Model file for the job. Use its own axes, mm. Give positions to 0.01 mm unless a question says otherwise; leave off trailing zeros. Write each loop counter-clockwise with the first axis right and the second up, starting at its lowest first coordinate (ties: lowest second). Pieces come first, ordered by that corner, then holes. Notation, with made-up numbers: (-2, -15) - (25, -15) arc R27 cw to (25, 16) - close; hole circle Ø2 at (65.25, 16). An arc over 180 degrees is marked (long way). One line per item, written item: value. Start each with the question number.
(1) Cut at C-C, the plane y = -51. List the corners of the cut face in (x, z).
(2) Cut at A-A, the plane x = 0.6. List the corners of the cut face in (y, z), and give its area (3 significant figures).
(3) Probe L1, parallel to Y at x = 1.9, z = -13; L2, parallel to Z at x = 2.15, y = -36.25; L3, parallel to Z at x = 1.9, y = -40.75. List the from-to ranges inside material, lowest first.
(4) Cut at B-B, the plane z = -15. List the corners of the cut face in (x, y).
(5) Drop flat-ended pins along their axis: P1, Ø0.8, axis at x = 1, z = -38, coming from the -Y side; P2, Ø0.8, axis at x = 1.5, y = -36, coming from the +Z side; P3, Ø1, axis at x = 0.5, z = -48.5, coming from the +Y side. Give the stop position or say it passes through.
from build123d import *

# Parameters (mm, degrees)
F1_DEPTH    = 2.54
F2_T1_DEPTH = 28.6682991577
F3_DEPTH    = 2.54
F4_DEPTH    = 2.54
F5_T1_DEPTH = 28.6682991577
F6_T1_DEPTH = 28.8815311919


# Not quite as in the source:
# - a fillet or chamfer that OpenCascade refuses, or shapes differently, is made with other operations: its cross-section is extruded or revolved along the edge and cut away or added


with BuildPart() as f1:
    # F0 (on Right) → F1 (new body)
    with BuildSketch(Plane.YZ):
        Polygon((-57.2273433208, -53.503472358), (-49.1374544799, -56.0896545649), (-49.1374544799, -53.503472358), align=None)
        Polygon((-49.1374544799, -53.503472358), (-49.1374544799, -56.0896545649), (-42.6720008254, -56.0896545649), (-42.6720008254, -53.503472358), (-42.6720008254, 0), (-49.1374544799, 0), align=None)
        with BuildLine():
            Line((-42.6720008254, -56.0896545649), (-49.1374544799, -56.0896545649))
            Line((-49.1374544799, -56.0896545649), (-49.1374544799, -67.4042031169))
            ThreePointArc((-49.1374544799, -67.4042031169), (-45.9047276527, -64.1714762896), (-42.6720008254, -67.4042031169))
            Line((-42.6720008254, -67.4042031169), (-42.6720008254, -56.0896545649))
        make_face()
        Polygon((-42.6720008254, -53.503472358), (-42.6720008254, -56.0896545649), (-33.620364964, -53.503472358), align=None)
        with BuildLine():
            ThreePointArc((-42.6720008254, -67.4042031169), (-45.9047276527, -70.6369299442), (-49.1374544799, -67.4042031169))
            Line((-49.1374544799, -67.4042031169), (-49.1374544799, -71.8398466706))
            Line((-49.1374544799, -71.8398466706), (-42.6720008254, -71.8398466706))
            Line((-42.6720008254, -71.8398466706), (-42.6720008254, -67.4042031169))
        make_face()
        with BuildLine():
            ThreePointArc((-42.6720008254, -67.4042031169), (-45.9047276527, -64.1714762896), (-49.1374544799, -67.4042031169))
            ThreePointArc((-49.1374544799, -67.4042031169), (-45.9047276527, -70.6369299442), (-42.6720008254, -67.4042031169))
        make_face()
    extrude(amount=F1_DEPTH)

    # F2: chamfer of 5.08 on 2 edges, made by hand

    # F2_s2 → F2_t1 (cut)
    with BuildSketch(Plane.YZ.offset(-13.0641495789)):
        Polygon((-44.0574544799, 0), (-49.1374544799, -5.08), (-49.1374544799, 0), align=None)
        Polygon((-42.6720008254, -5.08), (-47.7520008254, 0), (-42.6720008254, 0), align=None)
    extrude(amount=F2_T1_DEPTH, mode=Mode.SUBTRACT)

    # F0 (on Right) → F3 (join)
    with BuildSketch(Plane.YZ):
        Polygon((-57.2273433208, -53.503472358), (-49.1374544799, -56.0896545649), (-49.1374544799, -53.503472358), align=None)
        Polygon((-49.1374544799, -53.503472358), (-49.1374544799, -56.0896545649), (-42.6720008254, -56.0896545649), (-42.6720008254, -53.503472358), (-42.6720008254, 0), (-49.1374544799, 0), align=None)
        with BuildLine():
            Line((-42.6720008254, -56.0896545649), (-49.1374544799, -56.0896545649))
            Line((-49.1374544799, -56.0896545649), (-49.1374544799, -67.4042031169))
            ThreePointArc((-49.1374544799, -67.4042031169), (-45.9047276527, -64.1714762896), (-42.6720008254, -67.4042031169))
            Line((-42.6720008254, -67.4042031169), (-42.6720008254, -56.0896545649))
        make_face()
        Polygon((-42.6720008254, -53.503472358), (-42.6720008254, -56.0896545649), (-33.620364964, -53.503472358), align=None)
        with BuildLine():
            ThreePointArc((-42.6720008254, -67.4042031169), (-45.9047276527, -70.6369299442), (-49.1374544799, -67.4042031169))
            Line((-49.1374544799, -67.4042031169), (-49.1374544799, -71.8398466706))
            Line((-49.1374544799, -71.8398466706), (-42.6720008254, -71.8398466706))
            Line((-42.6720008254, -71.8398466706), (-42.6720008254, -67.4042031169))
        make_face()
        with BuildLine():
            ThreePointArc((-42.6720008254, -67.4042031169), (-45.9047276527, -64.1714762896), (-49.1374544799, -67.4042031169))
            ThreePointArc((-49.1374544799, -67.4042031169), (-45.9047276527, -70.6369299442), (-42.6720008254, -67.4042031169))
        make_face()
    extrude(amount=F3_DEPTH)

    # F0 (on Right) → F4 (join)
    with BuildSketch(Plane.YZ):
        Polygon((-57.2273433208, -53.503472358), (-49.1374544799, -56.0896545649), (-49.1374544799, -53.503472358), align=None)
        Polygon((-49.1374544799, -53.503472358), (-49.1374544799, -56.0896545649), (-42.6720008254, -56.0896545649), (-42.6720008254, -53.503472358), (-42.6720008254, 0), (-49.1374544799, 0), align=None)
        with BuildLine():
            Line((-42.6720008254, -56.0896545649), (-49.1374544799, -56.0896545649))
            Line((-49.1374544799, -56.0896545649), (-49.1374544799, -67.4042031169))
            ThreePointArc((-49.1374544799, -67.4042031169), (-45.9047276527, -64.1714762896), (-42.6720008254, -67.4042031169))
            Line((-42.6720008254, -67.4042031169), (-42.6720008254, -56.0896545649))
        make_face()
        Polygon((-42.6720008254, -53.503472358), (-42.6720008254, -56.0896545649), (-33.620364964, -53.503472358), align=None)
        with BuildLine():
            ThreePointArc((-42.6720008254, -67.4042031169), (-45.9047276527, -70.6369299442), (-49.1374544799, -67.4042031169))
            Line((-49.1374544799, -67.4042031169), (-49.1374544799, -71.8398466706))
            Line((-49.1374544799, -71.8398466706), (-42.6720008254, -71.8398466706))
            Line((-42.6720008254, -71.8398466706), (-42.6720008254, -67.4042031169))
        make_face()
        with BuildLine():
            ThreePointArc((-42.6720008254, -67.4042031169), (-45.9047276527, -64.1714762896), (-49.1374544799, -67.4042031169))
            ThreePointArc((-49.1374544799, -67.4042031169), (-45.9047276527, -70.6369299442), (-42.6720008254, -67.4042031169))
        make_face()
    extrude(amount=F4_DEPTH)

    # F5: chamfer of 5.08 on 2 edges, made by hand

    # F5_s2 → F5_t1 (cut)
    with BuildSketch(Plane.YZ.offset(-13.0641495789)):
        Polygon((-49.1374544799, -5.08), (-44.0574544799, 0), (-49.1374544799, 0), align=None)
        Polygon((-42.6720008254, -5.08), (-47.7520008254, 0), (-42.6720008254, 0), align=None)
    extrude(amount=F5_T1_DEPTH, mode=Mode.SUBTRACT)

    # F6: chamfer of 5.08 on 2 edges, made by hand

    # F6_s2 → F6_t1 (cut)
    with BuildSketch(Plane.YZ.offset(-13.170765596)):
        Polygon((-49.1374544799, -10.16), (-45.5453520315, -1.4878975516), (-49.1374544799, -5.08), align=None)
        Polygon((-46.2641032738, -1.4878975516), (-42.6720008254, -10.16), (-42.6720008254, -5.08), align=None)
    extrude(amount=F6_T1_DEPTH, mode=Mode.SUBTRACT)


solid = f1.part
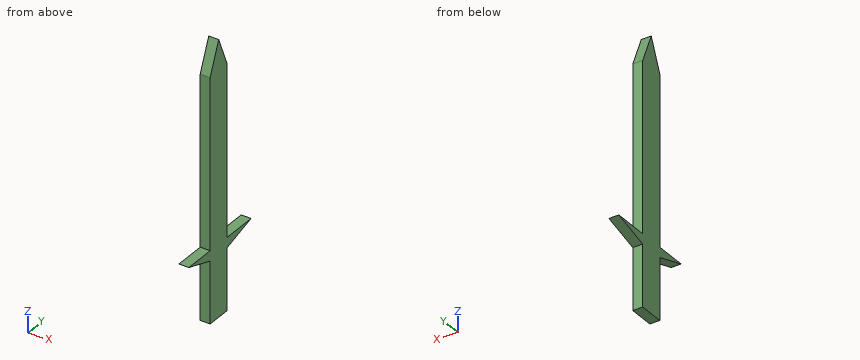
Answers follow:
1. outline: (0, -55.49) - (2.54, -55.49) - (2.54, -53.5) - (0, -53.5) - close
2. outline: (-57.23, -53.5) - (-49.14, -56.09) - (-49.14, -71.84) - (-42.67, -71.84) - (-42.67, -56.09) - (-33.62, -53.5) - (-42.67, -53.5) - (-42.67, -10.16) - (-45.9, -2.36) - (-49.14, -10.16) - (-49.14, -53.5) - close
2. area: 446 mm²
3. L1: y = -49.14 to -42.67
3. L2: z = -54.25 to -53.5
3. L3: z = -55.54 to -53.5
4. outline: (0, -49.14) - (2.54, -49.14) - (2.54, -42.67) - (0, -42.67) - close
5. P1: stops at y = -49.14
5. P2: stops at z = -53.5
5. P3: stops at y = -42.67
